Geometry: see drawing. Coordinates: mm, zero at the bounding-box minimum. A direction names the side the tool comes from. Round coordinates to 2 decimals unless told otherwise and drop trailing zeros. Write each loop counter-clockwise with the first axis right and the second up, starting at its lowest first coordinate (ties: lowest second). Pieces come first, ordered by that corner, then holes.
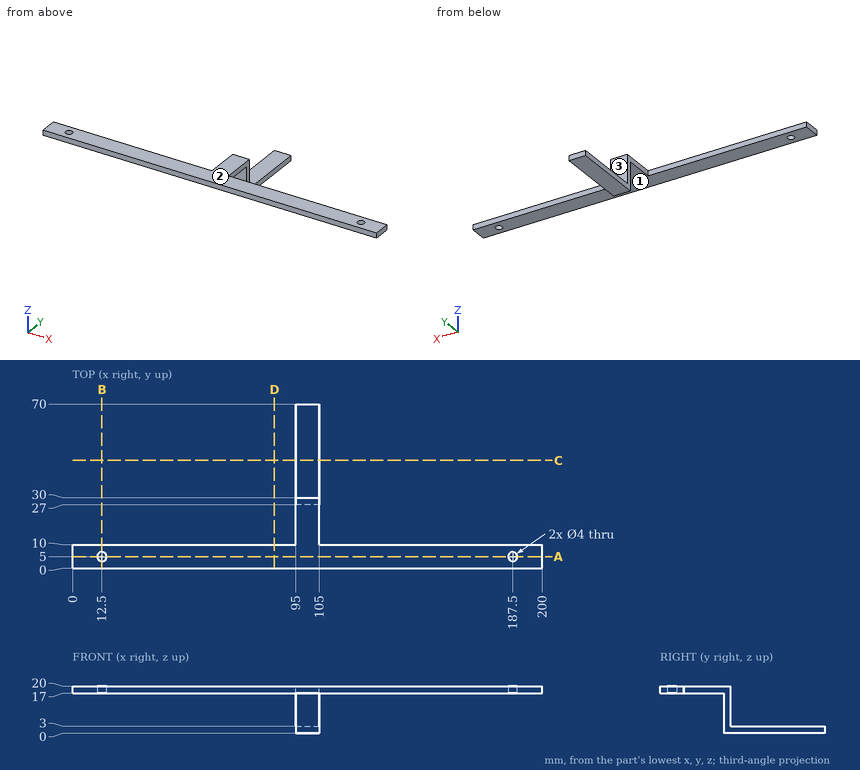
1) Section query D-D on x = 86. Return the cut outline in (y, z), then the cut area to 3 significant figures.
Taken from the geometry:
outline: (0, 17) - (10, 17) - (10, 20) - (0, 20) - close
area: 30.0 mm2
2) Contact query for flat-ended pins moving along their axis: P1, Ø3, axis at y = 43, z = 3.5, coming from the -X side; P2, Ø8, axis at y = 27.5, z = 18, coming from the +X side; P3, Ø11, axis at x = 98, z = 9.5, coming from the +Y side; P4, Ø12, axis at y = 52.5, z = 10.5, coming from the +X side. Output: stop coordinate, or through.
Taken from the geometry:
P1: stops at x = 95
P2: stops at x = 105
P3: stops at y = 30
P4: passes through
3) Reachability of the marked faces 1, 2 and 3 from +Z, -Z, +X, -X, +Y, -Y: full face, straight path, thin tool, end or side. Return the list, or none.
Taken from the geometry:
face 1: -Z, +X, -X, -Y
face 2: +Z, +X, -X, +Y, -Y
face 3: +Z, +X, -X, +Y
4) Section query A-A on y = 5. Return the cut outline in (x, z).
Taken from the geometry:
outline: (0, 17) - (10.5, 17) - (10.5, 20) - (0, 20) - close; (14.5, 17) - (185.5, 17) - (185.5, 20) - (14.5, 20) - close; (189.5, 17) - (200, 17) - (200, 20) - (189.5, 20) - close
5) Material intervals for line 1 (Y direction, x = 187.5, z = 19.05); line 2 (X direction, y = 38.5, z = 2.75); line 3 (Z direction, x = 134, y = 8), sorted ascending.
Taken from the geometry:
line 1: y = 0 to 3, 7 to 10
line 2: x = 95 to 105
line 3: z = 17 to 20
6) Section query C-C on y = 46. Return the cut outline in (x, z).
Taken from the geometry:
outline: (95, 0) - (105, 0) - (105, 3) - (95, 3) - close
7) Section query B-B on x = 12.5. Return the cut outline in (y, z).
Taken from the geometry:
outline: (0, 17) - (3, 17) - (3, 20) - (0, 20) - close; (7, 17) - (10, 17) - (10, 20) - (7, 20) - close
